Here's how the part is built. I have some questions about the finished solid (model axes, mm). A direction names the side the tool comes from. Give positions to 0.01 mm unless a question says otherwise; leave off trailing zeros. Write each loop counter-clockwise with the first axis right and the second up, starting at its lowest first coordinate (ties: lowest second). Pieces come first, ordered by that corner, then holes. Notation, with made-up numbers: (69, 22.5) -> (81, 22.5) arc R37 cw to (81, 61.5) -> close; hole circle Ø9 at (-26.75, 23). An arc over 180 degrees is marked (long way). Use CSV: the item, a comma, the result in double quotes. Start each with the question number.
(1) For pin 1 Ø5.5 at (x, z) = (4.5, 45) entering from +Y (3 decimals); pin 2 Ø3 at (y, z) = (40, 53.5) entering from +X (3 decimals); pin 3 Ø5 at (x, y) = (62.5, 10) entering from +Z (3 decimals); pin 4 Ø7.5 at (x, z) = (0, 66.2) entering from +Y, each with a flat end and sliding along its axis, tell me the tip position at first contact or that it passes through.
(2) Which directions (+Z, -Z, +X, -X, +Y, -Y) give clear straight access to the entire face, cutting with the end or side of a thin tool? Please do faces 1 (the flat face through (0, 41, 76.2)), 2 (the cylindrical face through (36.975, 19.444, 1.24)).
(3) Suppose I cut it at D-D on x = 7.5. List the corners of the cut face in (y, z) for me (3 decimals), plus the area to 3 significant figures.
(4) If we mould it in two halves opening along Y, with no side actions, what happens to faces 3 (the cylindrical face through (-9.3, 25.04, -2.06)), 4 (the flat face through (0, 43.975, 38)), 5 (the flat face through (75, 10, 0)), 6 (the flat face through (-8, 0, 4))? For each: pulls with the +Y half, pulls with the -Y half, needs draft (parallel to the pull), parting line crosses it, or undercut.
(5) Suppose I cut it at C-C on y = 40. Give the number of separate pieces and of enclosed holes in the cut face, plus the area to 3 significant figures.
(6) I need wall thicknesses on L1, parallel to X at y = 39, z = 66.2 (3 decimals); L2, parallel to X at y = 14.5, z = 0 (3 decimals); L3, parallel to Z at x = -3, y = 12.5. Which ranges of each line are inside material? Lowest first, please. Write a range as [from, to].
(7) Suppose I cut it at B-B on z = 66.2. List the corners of the cut face in (x, y) for me (3 decimals).
from build123d import *

# Parameters (mm, degrees)
SKETCH1_R          = 9.525
SLEEVE_DEPTH       = 50.8
SKETCH2_W          = 19.05
SKETCH2_H          = 6.35
BRACKET_DEPTH      = 76.2
SKETCH4_R          = 6.35
BRACKET_HOLE_DEPTH = 93.075
SKETCH5_R          = 9.525
SHAFT_DEPTH        = 75
SKETCH6_R          = 8.73125
SLEEVE_HOLE_DEPTH  = 119.372631972


with BuildPart() as part:
    # Sketch1 → Sleeve (new body)
    with BuildSketch(Plane(origin=(0, 0, 0), x_dir=(1, 0, 0), z_dir=(0, 1, 0))):
        with Locations(Location((0, 0, 0), (0, 0, 270))):
            Circle(SKETCH1_R)
    extrude(amount=SLEEVE_DEPTH)

    # Sketch2 → Bracket (add)
    with BuildSketch(Plane.XY):
        with Locations((0, 40.8)):
            Rectangle(SKETCH2_W, SKETCH2_H)
    extrude(amount=BRACKET_DEPTH)

    # Sketch4 → Bracket Hole (cut, through all)
    with BuildSketch(Plane(origin=(0, 0, 0), x_dir=(1, 0, 0), z_dir=(0, 1, 0))):
        with Locations(Location((0, -66.2, 0), (0, 0, 90))):
            Circle(SKETCH4_R)
    extrude(amount=BRACKET_HOLE_DEPTH, mode=Mode.SUBTRACT)

    # Sketch5 → Shaft (add)
    with BuildSketch(Plane(origin=(0, 0, 0), x_dir=(0, 0, -1), z_dir=(1, 0, 0))):
        with Locations((0, 10)):
            Circle(SKETCH5_R)
    extrude(amount=SHAFT_DEPTH)

    # Sketch6 → Sleeve Hole (cut, through all)
    with BuildSketch(Plane(origin=(0, 0, 0), x_dir=(1, 0, 0), z_dir=(0, 1, 0))):
        with Locations(Location((0, 0, 0), (0, 0, 270))):
            Circle(SKETCH6_R)
    extrude(amount=SLEEVE_HOLE_DEPTH, mode=Mode.SUBTRACT)


solid = part.part
Geometry says:
1,pin 1,"y = 43.975"
1,pin 2,"x = 9.525"
1,pin 3,"z = 9.525"
1,pin 4,"through"
2,face 1,"+Z, +X, -X, +Y, -Y"
2,face 2,"+X"
3,outline,"(0, -5.872) -> (2.5, -5.872) arc R9.525 ccw to (17.5, -5.872) -> (50.8, -5.872) -> (50.8, -4.47) -> (0, -4.47) -> close; (0, 4.47) -> (50.8, 4.47) -> (50.8, 5.872) -> (43.975, 5.872) -> (43.975, 76.2) -> (37.625, 76.2) -> (37.625, 5.872) -> (17.5, 5.872) arc R9.525 ccw to (2.5, 5.872) -> (0, 5.872) -> close"
3,area,"665 mm²"
4,face 3,"undercut"
4,face 4,"pulls with the +Y half"
4,face 5,"needs draft"
4,face 6,"pulls with the -Y half"
5,separate pieces,"1"
5,enclosed holes,"2"
5,area,"1,230 mm²"
6,L1,"[-9.525, -6.35], [6.35, 9.525]"
6,L2,"[-9.525, -8.731], [8.731, 75]"
6,L3,"[-9.04, -8.2], [8.2, 9.04]"
7,outline,"(-9.525, 37.625) -> (-6.35, 37.625) -> (-6.35, 43.975) -> (-9.525, 43.975) -> close; (6.35, 37.625) -> (9.525, 37.625) -> (9.525, 43.975) -> (6.35, 43.975) -> close"
